Can you work these out from the model? Positions are in its coordinate system, mm. A direction names the side the tool comes from. Coordinates: 2 decimals unless noted, no trailing zeros. Order: outer loops, then holes, each group sorted by start corner. A loop starts at its lowest first (then second) coordinate and runs counter-clockwise, first axis right, second up. Notation, with made-up numbers: (24.5, 2) -> (61.5, 2) arc R20 ccw to (61.5, 14) -> close; hole circle Ø8 at (15, 63.25). An arc over 180 degrees is marked (long way). Use a Markdown table: item, result. Add a question column.
1. Suppose I cut it at C-C, the plane z = 3. List the corners of the cut face in (x, y) for me (1 decimal), then the cut area to 3 significant figures.
2. Suppose I cut it at D-D, the plane x = 8.5. List the corners of the cut face in (y, z) for me.
3. Suppose I cut it at A-A, the plane z = 14. List the corners of the cut face in (x, y) for me (1 decimal), then the cut area to 3 significant figures.
4. If I drill on line 1 along X through (y, z) = (-1.5, 16); line 2 along Y through (x, z) = (-5, 9.5) (3 decimals); line 3 along Y through (x, z) = (9, 4.75), over which ranges is the centre line in solid material (lowest first)? Write a range as from..to.
5. Suppose I cut it at B-B, the plane y = -6.5. List the corners of the cut face in (x, z) for me, then the cut area to 3 significant figures.
6. We'd pull the mould along X, two halves only. Please class faces 1 (the flat face through (10, -5, 13)), 2 (the flat face through (30, -5, 13)), 3 (the flat face through (15, 0, 18)): pulls with the +X half, pulls with the -X half, needs draft (parallel to the pull), parting line crosses it, or undercut.
7. For faces 4 (the flat face through (20, -5, 13)), 5 (the cylindrical face through (1.737, -9.847, 12.675)), 6 (the cylindrical face through (26.99, -5.07, 2.85)), 7 (the flat face through (-11, 8, 25)), 8 (the flat face through (17, -10, 18)), which set-ups out of +Z, -Z, +X, -X, +Y, -Y let a thin tool reach every point of the face, with its end or its side?
8. For pin 1 Ø3 at (y, z) = (20, 3.5) entering from +X; pin 2 Ø12 at (x, z) = (-1, 5) entering from +Y; pin 3 Ø1.5 at (x, z) = (8, 3.5) entering from +Y, each with a flat end and sliding along its axis, tell me the tip position at first contact or that it passes through.
```python
from build123d import *

# Parameters (mm, degrees)
EXTRUDE_1_DEPTH     = 25
SKETCH_2_R          = 5
CUT_EXTRUDE_1_DEPTH = 58.049387676
SKETCH_6_W          = 30
SKETCH_6_H          = 25
EXTRUDE_2_DEPTH     = 10
SKETCH_7_W          = 10
SKETCH_7_H          = 10
CUT_EXTRUDE_2_DEPTH = 10
FILLET_1_R          = 10
FILLET_2_R          = 10


with BuildPart() as part:
    # 草图1 → 凸台-拉伸1 (new body)
    with BuildSketch(Plane.XY):
        with BuildLine():
            Line((-25, 31.224989992), (0, 0))
            ThreePointArc((0, 0), (-1.167185623, -10.542185623), (-11.709371247, -9.375))
            Line((-11.709371247, -9.375), (-36.709371247, 21.849989992))
            ThreePointArc((-36.709371247, 21.849989992), (-35.542185623, 32.392175615), (-25, 31.224989992))
        make_face()
    extrude(amount=EXTRUDE_1_DEPTH)

    # 草图2 → 切除-拉伸1 (cut, through all)
    with BuildSketch(Plane.XY.offset(25)):
        with Locations((-30.854685623, 26.537489992)):
            Circle(SKETCH_2_R)
        with Locations((-5.854685623, -4.6875)):
            Circle(SKETCH_2_R)
    extrude(amount=-CUT_EXTRUDE_1_DEPTH, mode=Mode.SUBTRACT)

    # 草图6 → 凸台-拉伸2 (add)
    with BuildSketch(Plane(origin=(0, 0, 0), x_dir=(1, 0, 0), z_dir=(0, 1, 0))):
        with Locations((15, -12.5)):
            Rectangle(SKETCH_6_W, SKETCH_6_H)
    extrude(amount=-EXTRUDE_2_DEPTH)

    # 草图7 → 切除-拉伸2 (cut)
    with BuildSketch(Plane(origin=(0, 0, 0), x_dir=(1, 0, 0), z_dir=(0, 1, 0))):
        with Locations((15, -12.5)):
            Rectangle(SKETCH_7_W, SKETCH_7_H)
    extrude(amount=-CUT_EXTRUDE_2_DEPTH, mode=Mode.SUBTRACT)

    # 圆角1
    fillet_1_edges = [part.edges().sort_by_distance(p)[0] for p in [
        (30, -5, 0),
        (30, -5, 25),
    ]]
    fillet(fillet_1_edges, radius=FILLET_1_R)

    # 圆角2
    # the kernel refuses this fillet: 10 mm, written as the material it takes off along each edge
    with BuildSketch(Plane(origin=(0, -10, 33.699631817), x_dir=(1, 0, 0), z_dir=(0, 0, -1))) as fillet_2_piece_1:
        with BuildLine():
            CenterArc((3.479852727, -10), FILLET_2_R, 90, 20.364134806)
            Line((0, -0.625), (-0.069597055, -0.4375))
            ThreePointArc((-0.069597055, -0.4375), (-0.2, -0.3125), (-0.2, 0))
            Line((-0.2, 0), (0, 0.2))
            Line((0, 0.2), (3.479852727, 0.2))
            Line((3.479852727, 0.2), (3.479852727, 0))
        make_face()
    extrude(amount=42.399263634, mode=Mode.SUBTRACT)


solid = part.part
```
Worked out:
| question | item | result |
|---|---|---|
| 1 | outline | (-36.7, 21.8) -> (-11.7, -9.4) arc R7.5 ccw to (0, -9.4) arc R10 ccw to (3.5, -10) -> (27.1, -10) -> (27.1, 0) -> (0, 0) -> (-25, 31.2) arc R7.5 ccw to start; hole circle Ø10 at (-30.9, 26.5); hole circle Ø10 at (-5.9, -4.7) |
| 1 | area | 880 mm² |
| 2 | outline | (-10, 0) -> (0, 0) -> (0, 25) -> (-10, 25) -> close |
| 3 | outline | (-36.7, 21.8) -> (-11.7, -9.4) arc R7.5 ccw to (0, -9.4) arc R10 ccw to (3.5, -10) -> (10, -10) -> (10, 0) -> (0, 0) -> (-25, 31.2) arc R7.5 ccw to start; (20, -10) -> (30, -10) -> (30, 0) -> (20, 0) -> close; hole circle Ø10 at (-30.9, 26.5); hole circle Ø10 at (-5.9, -4.7) |
| 3 | area | 808 mm² |
| 4 | line 1 | x = -18.01..-9.71, -2..10, 20..29.95 |
| 4 | line 2 | y = -12.139..-9.614, 0.239..6.245 |
| 4 | line 3 | y = -10..0 |
| 5 | outline | (-14.01, 0) -> (-10.51, 0) -> (-10.51, 25) -> (-14.01, 25) -> close; (-1.19, 0) -> (20, 0) arc R10 ccw to (30, 10) -> (30, 15) arc R10 ccw to (20, 25) -> (-1.19, 25) -> close; hole (10, 7.5) -> (20, 7.5) -> (20, 17.5) -> (10, 17.5) -> close |
| 5 | area | 724 mm² |
| 6 | face 1 | undercut |
| 6 | face 2 | pulls with the +X half |
| 6 | face 3 | needs draft |
| 7 | face 4 | +Y, -Y |
| 7 | face 5 | +Z, -Z, -Y |
| 7 | face 6 | -Z, +X, +Y, -Y |
| 7 | face 7 | +Z, +X, -X, +Y, -Y |
| 7 | face 8 | +Z, -Z, +X, -Y |
| 8 | pin 1 | stops at x = -14.81 |
| 8 | pin 2 | stops at y = 8.74 |
| 8 | pin 3 | stops at y = 0 |
